Source: CAD feature listing. Evaluate the final solid. Frame: model axes, mm. A direction names the side the tool comes from. Give positions to 0.01 mm unless a question says otherwise; leave off trailing zeros. Loops run counter-clockwise (first coordinate to the right, second up) from the corner with the lowest first, then second, coordinate; pieces in that order, holes last. Notation, with made-up numbers: (32.25, 59.25) -> (81.25, 59.25) arc R27 cw to (81.25, 92.25) -> close; hole circle Ø2 at (-18, 39.5). An arc over 180 degrees is marked (long way). Return JSON: item names as keys, results as strings. Group by question number.
```python
from build123d import *

# Parameters (mm, degrees)
F0_W      = 30
F0_H      = 30
F1_DEPTH  = 11
F2_W      = 26
F2_H      = 30
F3_DEPTH  = 9
F4_W      = 1.45
F4_H      = 30
F5_DEPTH  = 9
F5_FACE_W = 10.1
F5_FACE_H = 30
F6_DEPTH  = 4
F7_W      = 3.5
F7_H      = 2.5
F8_DEPTH  = 13


with BuildPart() as f1:
    # F0 (on Top) → F1 (new body)
    with BuildSketch(Plane.XY):
        Rectangle(F0_W, F0_H)
    extrude(amount=F1_DEPTH)

    # F2 (on face) → F3 (cut)
    with BuildSketch(Plane(origin=(0, 0, 0), x_dir=(1, 0, 0), z_dir=(0, 0, -1))):
        Rectangle(F2_W, F2_H)
    extrude(amount=-F3_DEPTH, mode=Mode.SUBTRACT)

    # F4 (on face) → F5 (join)
    with BuildSketch(Plane.XY.offset(11)):
        with Locations((-5.775, 0)):
            Rectangle(F4_W, F4_H)
        with Locations((5.775, 0)):
            Rectangle(F4_W, F4_H)
    extrude(amount=F5_DEPTH)

    # F5_face (on face) → F6 (join)
    with BuildSketch(Plane.XY.offset(11)):
        Rectangle(F5_FACE_W, F5_FACE_H)
    extrude(amount=F6_DEPTH)

    # F7 (on face) → F8 (cut, through all)
    with BuildSketch(Plane.YZ.offset(6.5)):
        with Locations((-8.25, 12.25)):
            Rectangle(F7_W, F7_H)
        with Locations((8.25, 12.25)):
            Rectangle(F7_W, F7_H)
    extrude(amount=-F8_DEPTH, mode=Mode.SUBTRACT)


solid = f1.part
```
1) Cut plane D-D on y = -6. Return loops of the section in (x, z).
2) Material intervals for line 1 (X direction, y = 1.5, z = 8.75); line 2 (X direction, y = 13, z = 18.5); line 3 (Z direction, x = -2.5, y = 7), sorted ascending.
3) Mould query, pull axis Z, two halves, no side actions, for faces 5 (the face through (-14, 0, 0)), 6 (the face through (-6, 0, 20)), 7 (the face through (0, 8, 13.5)). Classes: released by +Z, released by -Z, zero draft, split by the parting line, or undercut.
4) Reachability of faces 1 (the face through (0, 0, 15)), 2 (the face through (13, 0, 4)), 3 (the face through (-7, 0, 11)), 4 (the face through (0, 10, 12)) from +Z, -Z, +X, -X, +Y, -Y: full face, straight path, thin tool, end or side. Return the list, or none.
5) Cut plane B-B on y = 7.25. Return loops of the section in (x, z).
6) Contact query for flat-ended pins moving along their axis: P1, Ø6, axis at x = -1.5, y = -10, coming from the +Z side; P2, Ø2.5, axis at y = 4, z = 16.5, coming from the +X side; P3, Ø1.8, axis at x = -1.5, y = -9, coming from the -Z side; P4, Ø8, axis at x = 5, y = -1.5, coming from the +Z side. Output: stop coordinate, or through.
7) Cut plane A-A on z = 8.5. Return loops of the section in (x, y).
8) Cut plane C-C on x = 2.75. Return loops of the section in (y, z).
Calculated:
{
 "1": {"outline": "(-15, 0) -> (-13, 0) -> (-13, 9) -> (13, 9) -> (13, 0) -> (15, 0) -> (15, 11) -> (6.5, 11) -> (6.5, 20) -> (5.05, 20) -> (5.05, 15) -> (-5.05, 15) -> (-5.05, 20) -> (-6.5, 20) -> (-6.5, 11) -> (-15, 11) -> close"},
 "2": {"line 1": "-15 to -13, 13 to 15", "line 2": "-6.5 to -5.05, 5.05 to 6.5", "line 3": "9 to 11, 13.5 to 15"},
 "3": {"face 5": "released by -Z", "face 6": "released by +Z", "face 7": "undercut"},
 "4": {"face 1": "+Z, +Y, -Y", "face 2": "-Z, +Y, -Y", "face 3": "none", "face 4": "+X, -X"},
 "5": {"outline": "(-15, 0) -> (-13, 0) -> (-13, 9) -> (13, 9) -> (13, 0) -> (15, 0) -> (15, 11) -> (-15, 11) -> close; (-6.5, 13.5) -> (6.5, 13.5) -> (6.5, 20) -> (5.05, 20) -> (5.05, 15) -> (-5.05, 15) -> (-5.05, 20) -> (-6.5, 20) -> close"},
 "6": {"P1": "z = 15", "P2": "x = 6.5", "P3": "z = 9", "P4": "z = 20"},
 "7": {"outline": "(-15, -15) -> (-13, -15) -> (-13, 15) -> (-15, 15) -> close; (13, -15) -> (15, -15) -> (15, 15) -> (13, 15) -> close"},
 "8": {"outline": "(-15, 9) -> (15, 9) -> (15, 15) -> (-15, 15) -> close; hole (-10, 11) -> (-6.5, 11) -> (-6.5, 13.5) -> (-10, 13.5) -> close; hole (6.5, 11) -> (10, 11) -> (10, 13.5) -> (6.5, 13.5) -> close"}
}
